Can you work these out from the model? Positions are in its coordinate system, mm. Give positions to 0.01 mm unless a question says otherwise; leave off trailing zeros. Order: outer loops, then holes, each group sorted by start corner. A loop starts at its lowest first (then second) coordinate and runs counter-clockwise, first axis right, second up. Notation, with made-up numbers: (45.5, 63) -> (54.5, 63) arc R9 cw to (54.5, 80) -> close; hole circle Ø10 at (33, 73.5). An arc over 180 degrees is marked (long way). Answer as a JSON object with one key per item and string values.
```python
from build123d import *

# Parameters (mm, degrees)
BASE_FLANGE1_DEPTH             = 170
EDGE_FLANGE1_STRIP_W           = 0.762
EDGE_FLANGE1_STRIP_H           = 0.127
EDGE_FLANGE1_STRIP_CUT_DEPTH   = 249.873
EDGE_FLANGE1_STRIP_2_W         = 0.762
EDGE_FLANGE1_STRIP_2_H         = 0.127
EDGE_FLANGE1_STRIP_CUT_2_DEPTH = 249.873
EDGE_FLANGE1_DEPTH             = 249.873
EDGE_FLANGE1_BEND_DEPTH        = 249.873
SKETCH19_W                     = 16
SKETCH19_H                     = 60
CUT_EXTRUDE1_DEPTH             = 10
SKETCH20_R                     = 1.5
CUT_EXTRUDE2_DEPTH             = 10


# Sheet-metal steps are written as plain solids
with BuildPart() as part:
    # Sketch1 → Base-Flange1 (new body)
    with BuildSketch(Plane.XY):
        with BuildLine():
            Line((0, 0), (249.873, 0))
            ThreePointArc((249.873, 0), (249.962802561, 0.037197439), (250, 0.127))
            Line((250, 0.127), (250, 7))
            Line((250, 7), (250.127, 7))
            Line((250.127, 7), (250.127, 0.127))
            ThreePointArc((250.127, 0.127), (250.052605122, -0.052605122), (249.873, -0.127))
            Line((249.873, -0.127), (0, -0.127))
            Line((0, -0.127), (0, 0))
        make_face()
    extrude(amount=BASE_FLANGE1_DEPTH)

    # Edge-Flange1 strip (across the edge) → Edge-Flange1 strip cut (cut)
    with BuildSketch(Plane.ZY.offset(-249.873)):
        with Locations((-0.127, -0.0635)):
            Rectangle(EDGE_FLANGE1_STRIP_W, EDGE_FLANGE1_STRIP_H)
    extrude(amount=EDGE_FLANGE1_STRIP_CUT_DEPTH, mode=Mode.SUBTRACT)

    # Edge-Flange1 strip 2 (across the edge) → Edge-Flange1 strip cut 2 (cut)
    with BuildSketch(Plane(origin=(0, 0, 170), x_dir=(0, 0, -1), z_dir=(1, 0, 0))):
        with Locations((-0.127, -0.0635)):
            Rectangle(EDGE_FLANGE1_STRIP_2_W, EDGE_FLANGE1_STRIP_2_H)
    extrude(amount=EDGE_FLANGE1_STRIP_CUT_2_DEPTH, mode=Mode.SUBTRACT)

    # Edge-Flange1 section (across the edge) → Edge-Flange1 (add)
    with BuildSketch(Plane.ZY.offset(-249.873)):
        with BuildLine():
            Line((0, 0.127), (0, 6.873))
            Line((0, 6.873), (0.127, 6.873))
            Line((0.127, 6.873), (0.127, 0.127))
            ThreePointArc((0.127, 0.127), (0.164197439, 0.037197439), (0.254, 0))
            Line((0.254, 0), (0.254, -0.127))
            ThreePointArc((0.254, -0.127), (0.074394878, -0.052605122), (0, 0.127))
        make_face()
    extrude(amount=EDGE_FLANGE1_DEPTH)

    # Edge-Flange1 section 2 (across the edge) → Edge-Flange1 bend (add)
    with BuildSketch(Plane(origin=(0, 0, 170), x_dir=(0, 0, -1), z_dir=(1, 0, 0))):
        with BuildLine():
            Line((0, 0.127), (0, 6.873))
            Line((0, 6.873), (0.127, 6.873))
            Line((0.127, 6.873), (0.127, 0.127))
            ThreePointArc((0.127, 0.127), (0.164197439, 0.037197439), (0.254, 0))
            Line((0.254, 0), (0.254, -0.127))
            ThreePointArc((0.254, -0.127), (0.074394878, -0.052605122), (0, 0.127))
        make_face()
    extrude(amount=EDGE_FLANGE1_BEND_DEPTH)

    # Sketch19 → Cut-Extrude1 (cut)
    with BuildSketch(Plane(origin=(0, 0, 0), x_dir=(1, 0, 0), z_dir=(0, 1, 0))):
        with Locations((8, -120.873)):
            Rectangle(SKETCH19_W, SKETCH19_H)
    extrude(amount=-CUT_EXTRUDE1_DEPTH, mode=Mode.SUBTRACT)

    # Sketch20 → Cut-Extrude2 (cut)
    with BuildSketch(Plane.ZY.offset(-250)):
        with Locations((30, 3.694801823)):
            Circle(SKETCH20_R)
        with Locations((140, 3.694801823)):
            Circle(SKETCH20_R)
    extrude(amount=-CUT_EXTRUDE2_DEPTH, mode=Mode.SUBTRACT)


solid = part.part
```
1. If we section it at C-C on z = 119.5: Please give me the cut outline in (x, y), then the cut area to 3 significant figures.
Worked answers:
{"outline": "(16, -0.13) -> (249.87, -0.13) arc R0.25 ccw to (250.13, 0.13) -> (250.13, 7) -> (250, 7) -> (250, 0.13) arc R0.13 cw to (249.87, 0) -> (16, 0) -> close", "area": "30.6 mm²"}
2. If we section it at B-B on z = 157.5: Please give me the cut outline in (x, y).
Worked answers:
{"outline": "(0, -0.13) -> (249.87, -0.13) arc R0.25 ccw to (250.13, 0.13) -> (250.13, 7) -> (250, 7) -> (250, 0.13) arc R0.13 cw to (249.87, 0) -> (0, 0) -> close"}
3. Will these pins go through, and if not, where does the flat tip stop? pin 1 Ø1.5 at (x, z) = (50, 82) entering from +Y; pin 2 Ø1.5 at (y, z) = (5.5, 111.5) entering from -X.
Worked answers:
{"pin 1": "y = 0", "pin 2": "x = 250"}
4. Please list where this line runs through material, in increasing order: L1, parallel to Y at x = 250.05, z = 140.
Worked answers:
{"L1": "-0.06 to 2.19, 5.19 to 7"}
5. If we section it at A-A on x = 108: Please give me the cut outline in (y, z), then the cut area to 3 significant figures.
Worked answers:
{"outline": "(-0.13, 0.25) arc R0.25 ccw to (0.13, 0) -> (6.87, 0) -> (6.87, 0.13) -> (0.13, 0.13) arc R0.13 cw to (0, 0.25) -> (0, 169.75) arc R0.13 cw to (0.13, 169.87) -> (6.87, 169.87) -> (6.87, 170) -> (0.13, 170) arc R0.25 ccw to (-0.13, 169.75) -> close", "area": "23.3 mm²"}
